from build123d import *

# Parameters (mm, degrees)
SKETCH1_W           = 214
SKETCH1_H           = 376
BOSS_EXTRUDE1_DEPTH = 50.8
BOSS_EXTRUDE2_START = -50.8
SKETCH2_W           = 214
SKETCH2_H           = 325.2
BOSS_EXTRUDE2_DEPTH = 316


with BuildPart() as part:
    # Sketch1 → Boss-Extrude1 (new body)
    with BuildSketch(Plane(origin=(0, 0, 0), x_dir=(1, 0, 0), z_dir=(0, 1, 0))):
        Rectangle(SKETCH1_W, SKETCH1_H)
    extrude(amount=BOSS_EXTRUDE1_DEPTH)

    # Sketch2 → Boss-Extrude2 (add)
    with BuildSketch(Plane(origin=(0, 50.8, 0), x_dir=(1, 0, 0), z_dir=(0, 1, 0)).offset(BOSS_EXTRUDE2_START)):
        with Locations((0, 25.4)):
            Rectangle(SKETCH2_W, SKETCH2_H)
    extrude(amount=BOSS_EXTRUDE2_DEPTH)


solid = part.part
Input: part model. Units: mm. Frame: model coordinates. A direction names the side the tool comes from. Give positions to 0.01 mm unless a question says otherwise; leave off trailing zeros. Order: outer loops, then holes, each group sorted by start corner. A loop starts at its lowest first (then second) coordinate and runs counter-clockwise, first axis right, second up. Notation, with made-up numbers: M -4.5,48 L 40.5,48 A30 cw 40.5,71 Z; hole C 30.5,39.5 d5. An arc over 180 degrees is marked long. Answer as a JSON object with one key per item and string values.
1. First-contact query: P1, Ø1.5, axis at x = -5.5, y = 93, coming from the +Z side. Flat tip, straight axial feed; report the tip coordinate or a pass-through.
Result sheet:
{"P1": "z = 137.2"}
2. Reachability of faces 1 (the flat face through (-1, 316, -28)), 2 (the flat face through (-1, 182, 137.2)) from +Z, -Z, +X, -X, +Y, -Y: full face, straight path, thin tool, end or side. Return the list, or none.
Result sheet:
{"face 1": "+Z, -Z, +X, -X, +Y", "face 2": "+Z, +X, -X, +Y"}
3. Cut plane B-B, the plane y = 72.5. Output: boundary loops of the cut face in (x, z), and give its area (3 significant figures).
Result sheet:
{"outline": "M -107,-188 L 107,-188 L 107,137.2 L -107,137.2 Z", "area": "69,600 mm²"}
4. Ray query, line 1 (Z direction, x = 22.5, y = 178); line 2 (Y direction, x = -55, z = 168.5). Return the intervals inside material, ascending. Write a range as [from, to].
Result sheet:
{"line 1": "[-188, 137.2]", "line 2": "[0, 50.8]"}
5. Cut plane A-A, the plane x = 76. Output: boundary loops of the cut face in (y, z).
Result sheet:
{"outline": "M 0,-188 L 316,-188 L 316,137.2 L 50.8,137.2 L 50.8,188 L 0,188 Z"}
